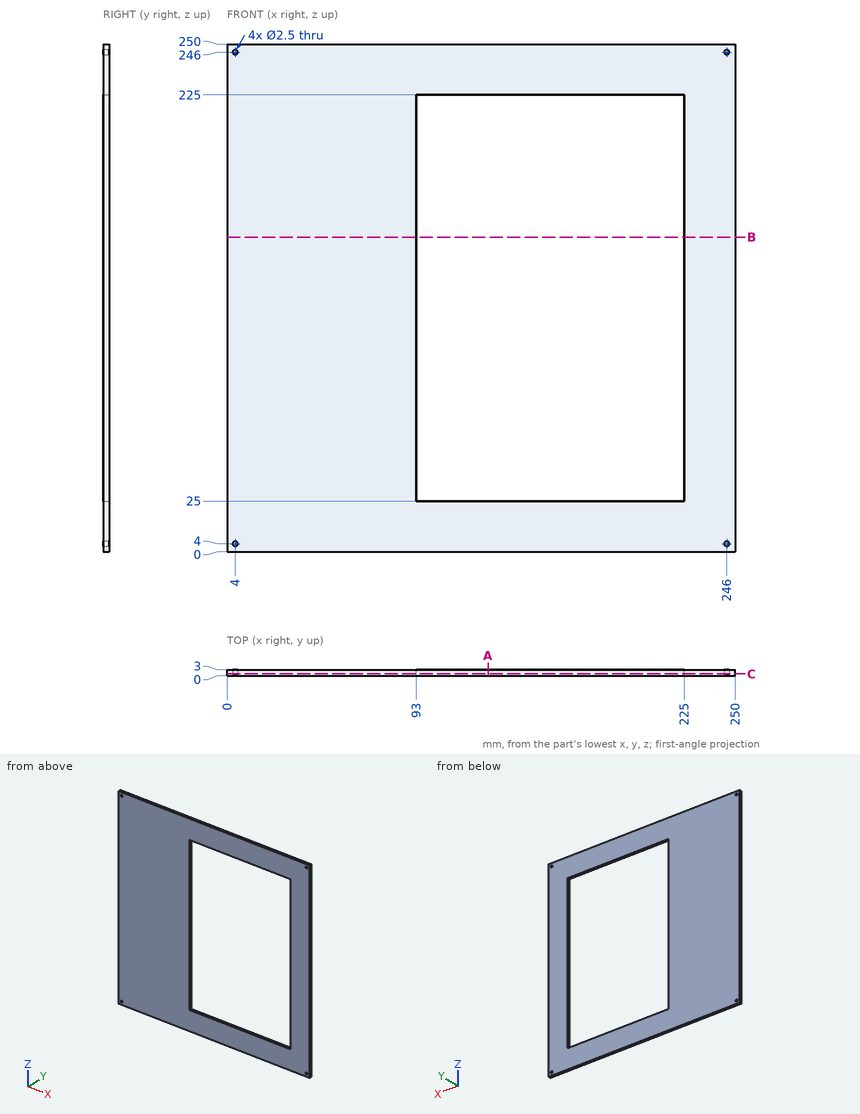
Job drawing, mm, ordinate dimensions from the low corner. One solid piece. Round coordinates to 2 decimals unless told otherwise and drop trailing zeros. Write each loop counter-clockwise with the first axis right and the second up, starting at its lowest first coordinate (ties: lowest second). Pieces come first, ordered by that corner, then holes.
1) Pin check, flat tip, straight feed: pin 1 (2 mm diameter, centred on x = 246, z = 4, fed in from +Y). Stop position of the tip, or through.
2) Band-saw the part on C-C, the plane y = 1. List the corners of the cut face in (x, z).
3) Band-saw the part on A-A, the plane x = 128.5. List the corners of the cut face in (y, z), and give its area (3 significant figures).
4) Drill centre lines: probe 1 along Z at (x, y) = (246, 1.3); probe 2 along Z at (x, y) = (158, 1.4). Where is each one in solid material? Low to high.
5) Band-saw the part on B-B, the plane z = 155. List the corners of the cut face in (x, y).
Ans:
1. pin 1: passes through
2. outline: (0, 0) - (250, 0) - (250, 250) - (0, 250) - close; hole circle Ø2.5 at (4, 4); hole circle Ø2.5 at (4, 246); hole (93, 25) - (225, 25) - (225, 225) - (93, 225) - close; hole circle Ø2.5 at (246, 4); hole circle Ø2.5 at (246, 246)
3. outline: (0, 0) - (3, 0) - (3, 25) - (0, 25) - close; (0, 225) - (3, 225) - (3, 250) - (0, 250) - close
3. area: 150 mm2
4. probe 1: z = 0 to 2.75, 5.25 to 244.75, 247.25 to 250
4. probe 2: z = 0 to 25, 225 to 250
5. outline: (0, 0) - (93, 0) - (93, 3) - (0, 3) - close; (225, 0) - (250, 0) - (250, 3) - (225, 3) - close
